Read the model definition and answer for the solid it produces. Units are mm, in the model's axes. Face numbers are marked on the shaded views. A direction names the side the tool comes from. Round coordinates to 2 decimals unless told otherwise and drop trailing zeros. Order: outer loops, then holes, each group sorted by start corner. A loop starts at its lowest first (then second) coordinate and runs counter-clockwise, first axis right, second up. Notation, with made-up numbers: (-15, 4) -> (3, 4) arc R12 ccw to (3, 8) -> close; hole circle Ø4 at (-38.75, 80). An arc over 180 degrees is marked (long way). One line per item, written item: value. Start each with the question number.
1. For the marked faces 1, 2 and 3, determine the directions among +Z, -Z, +X, -X, +Y, -Y from which every point of the face is accessible in a straight line to the end or side of a thin tool.
2. The mould has two halves that part along Y. Classify the marked faces 4, 5, 6 and 7: released by +Y, released by -Y, zero draft, split by the parting line, or undercut.
3. Section A-A (x = 14.5) is taken. Give the vertices of the cut face in (y, z), then the cut area to 3 significant figures.
4. Flat-ended cylindrical pins translate along their axes: pin 1 Ø1.2 at (y, z) = (0, 0) entering from -X; pin 2 Ø1 at (x, y) = (9.5, -2.5) entering from +Z; pin 3 Ø1.5 at (x, y) = (14, 3) entering from +Z. Find the tip coordinate at first contact, or state that the pin passes through.
5. Consider line 1 (Y direction, x = 9.5, z = 0.75); line 2 (Y direction, x = -6.15, z = 0) (3 decimals); line 3 (Y direction, x = 0, z = 0). Determine where each line is inside the solid, lowest interval first.
6. Section C-C (y = -6) is taken. Give the vertices of the cut face in (x, z), then the cut area to 3 significant figures.
7. Section D-D (z = -3.25) is taken. State how many separate pieces and enclosed holes the cut face has, then the cut area to 3 significant figures.
8. Section B-B (x = -3.75) is taken. Give the vertices of the cut face in (y, z) (3 decimals), then the cut area to 3 significant figures.
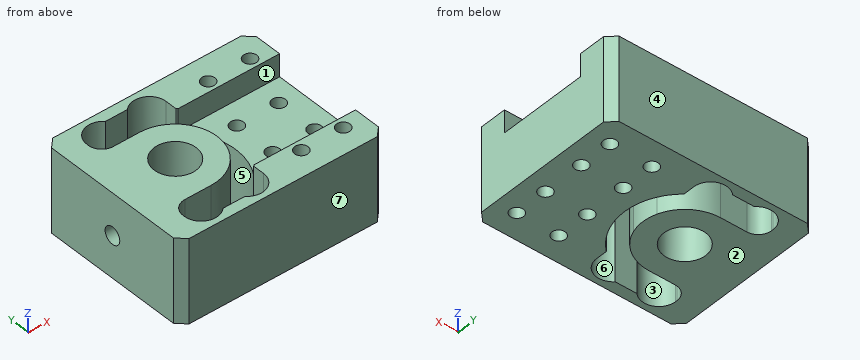
from build123d import *

# Parameters (mm, degrees)
SKETCH1_W                = 15
SKETCH1_H                = 19
BOSS_EXTRUDE1_DEPTH      = 5
BOSS_EXTRUDE1_DEPTH_BACK = 5
CUT_EXTRUDE1_START       = -6
SKETCH2_R                = 2
CUT_EXTRUDE1_DEPTH       = 16
SKETCH5_R                = 2
CUT_EXTRUDE4_DEPTH       = 17
CUT_EXTRUDE4_DEPTH_BACK  = 17
SKETCH6_R                = 2
CUT_EXTRUDE5_DEPTH       = 17
CUT_EXTRUDE5_DEPTH_BACK  = 17
SKETCH10_W               = 9.46
SKETCH10_H               = 13.6
CUT_EXTRUDE6_DEPTH       = 6
CUT_EXTRUDE6_DEPTH_BACK  = 6
BOSS_EXTRUDE2_START      = -5
SKETCH7_R                = 5
SKETCH7_R_2              = 2.5
BOSS_EXTRUDE2_DEPTH      = 10
BOSS_EXTRUDE3_DEPTH      = 5
FILLET1_R                = 1.6
SKETCH11_W               = 12.27
SKETCH11_H               = 19
BOSS_EXTRUDE4_DEPTH      = 10
CHAMFER1_SIZE            = 1
SKETCH16_W               = 5.80562201
SKETCH16_H               = 3.2
CUT_EXTRUDE8_DEPTH       = 11.5
CUT_EXTRUDE9_DEPTH       = 11.5
CUT_EXTRUDE10_DEPTH      = 2.7
TROU_TARAUD_M21_D        = 1.6
TROU_TARAUD_M2_51_D      = 2.05
TROU_TARAUD_M2_51_DEPTH  = 8.25
TROU_TARAUD_M2_51_TIP    = 0.615882135


with BuildPart() as part:
    # Sketch1 → Boss-Extrude1 (new body, two sides)
    with BuildSketch(Plane.XY) as boss_extrude1_sk:
        Rectangle(SKETCH1_W, SKETCH1_H)
    extrude(amount=BOSS_EXTRUDE1_DEPTH)
    extrude(boss_extrude1_sk.sketch, amount=-BOSS_EXTRUDE1_DEPTH_BACK)

    # Sketch2 → Cut-Extrude1 (cut)
    with BuildSketch(Plane.XY.offset(CUT_EXTRUDE1_START)):
        with Locations((-2.73, 6.8)):
            Circle(SKETCH2_R)
    cut_extrude1 = extrude(amount=CUT_EXTRUDE1_DEPTH, mode=Mode.SUBTRACT)

    # Mirror3: Cut-Extrude1 across plane
    add(cut_extrude1.mirror(Plane.ZX), mode=Mode.SUBTRACT)

    # Sketch5 → Cut-Extrude4 (cut, two sides)
    with BuildSketch(Plane.XY) as cut_extrude4_sk:
        with Locations((2.73, 6.8)):
            Circle(SKETCH5_R)
    extrude(amount=CUT_EXTRUDE4_DEPTH, mode=Mode.SUBTRACT)
    extrude(cut_extrude4_sk.sketch, amount=-CUT_EXTRUDE4_DEPTH_BACK, mode=Mode.SUBTRACT)

    # Sketch6 → Cut-Extrude5 (cut, two sides)
    with BuildSketch(Plane.XY) as cut_extrude5_sk:
        with Locations((2.73, -6.8)):
            Circle(SKETCH6_R)
    extrude(amount=CUT_EXTRUDE5_DEPTH, mode=Mode.SUBTRACT)
    extrude(cut_extrude5_sk.sketch, amount=-CUT_EXTRUDE5_DEPTH_BACK, mode=Mode.SUBTRACT)

    # Sketch10 → Cut-Extrude6 (cut, two sides)
    with BuildSketch(Plane.XY) as cut_extrude6_sk:
        Rectangle(SKETCH10_W, SKETCH10_H)
    extrude(amount=CUT_EXTRUDE6_DEPTH, mode=Mode.SUBTRACT)
    extrude(cut_extrude6_sk.sketch, amount=-CUT_EXTRUDE6_DEPTH_BACK, mode=Mode.SUBTRACT)



with BuildPart() as body_2:
    # Sketch7 → Boss-Extrude2 (new body)
    with BuildSketch(Plane.XY.offset(BOSS_EXTRUDE2_START)):
        Circle(SKETCH7_R)
        Circle(SKETCH7_R_2, mode=Mode.SUBTRACT)
    extrude(amount=BOSS_EXTRUDE2_DEPTH)


with BuildPart() as part_1:
    add(part.part)

    add(body_2.part)  # Boss-Extrude3 merges body 2
    # Sketch8 → Boss-Extrude3 (add, symmetric)
    with BuildSketch(Plane.XY):
        Polygon((0, 5), (-7.5, 5), (-7.5, 0), (-5, 0), align=None)
    boss_extrude3 = extrude(amount=BOSS_EXTRUDE3_DEPTH, both=True)

    # Mirror7: Boss-Extrude3 across plane
    add(boss_extrude3.mirror(Plane.ZX))

    # Fillet1
    fillet1_edges = [part_1.edges().sort_by_distance(p)[0] for p in [
        (-4.73, -5, 0),
        (-4.73, 5, 0),
    ]]
    fillet(fillet1_edges, radius=FILLET1_R)

    # Sketch11 → Boss-Extrude4 (add)
    with BuildSketch(Plane.XY.offset(5)):
        with Locations((10.865, 0)):
            Rectangle(SKETCH11_W, SKETCH11_H)
    extrude(amount=-BOSS_EXTRUDE4_DEPTH)

    # Chamfer1
    chamfer1_edges = [part_1.edges().sort_by_distance(p)[0] for p in [
        (17, 9.5, 0),
        (17, -9.5, 0),
        (-7.5, 9.5, 0),
        (-7.5, -9.5, 0),
    ]]
    chamfer(chamfer1_edges, length=CHAMFER1_SIZE)

    # Sketch16 → Cut-Extrude8 (cut)
    with BuildSketch(Plane.XY.offset(5)):
        with Locations((-0.227188995, 6.6)):
            Rectangle(SKETCH16_W, SKETCH16_H)
    cut_extrude8 = extrude(amount=-CUT_EXTRUDE8_DEPTH, mode=Mode.SUBTRACT)

    # Mirror8: Cut-Extrude8 across plane
    add(cut_extrude8.mirror(Plane.ZX), mode=Mode.SUBTRACT)

    # Sketch17 → Cut-Extrude9 (cut)
    with BuildSketch(Plane.XY.offset(5)):
        with BuildLine():
            ThreePointArc((2.678170763, -4.222250746), (5, 0), (2.678170763, 4.222250746))
            ThreePointArc((2.678170763, 4.222250746), (2.338473166, 5.740343478), (3.856565898, 6.080041075))
            ThreePointArc((3.856565898, 6.080041075), (7.2, 0), (3.856565898, -6.080041075))
            ThreePointArc((3.856565898, -6.080041075), (2.338473166, -5.740343478), (2.678170763, -4.222250746))
        make_face()
    extrude(amount=-CUT_EXTRUDE9_DEPTH, mode=Mode.SUBTRACT)

    # Sketch20 → Cut-Extrude10 (cut)
    with BuildSketch(Plane.XY.offset(5)):
        with BuildLine():
            Line((17, 5.3), (4.73, 5.3))
            ThreePointArc((4.73, 5.3), (7.103724375, 0), (4.73, -5.3))
            Line((4.73, -5.3), (17, -5.3))
            Line((17, -5.3), (17, 5.3))
        make_face()
    extrude(amount=-CUT_EXTRUDE10_DEPTH, mode=Mode.SUBTRACT)

    # Trou taraudé M21 (through all)
    with Locations(Plane.XY.offset(5)):
        with Locations((14.5, 2.5), (14.5, -2.5), (9.5, 2.5), (9.5, -2.5), (9.5, 6.5), (14.5, 6.5), (9.5, -6.5), (14.5, -6.5)):
            Hole(TROU_TARAUD_M21_D / 2)

    # Trou taraudé M2.51
    with Locations(Plane.ZY.offset(7.5)):
        with Locations((0, 0)):
            Hole(TROU_TARAUD_M2_51_D / 2, depth=TROU_TARAUD_M2_51_DEPTH)
            with Locations((0, 0, -(TROU_TARAUD_M2_51_DEPTH + TROU_TARAUD_M2_51_TIP / 2))):  # 118° drill point
                Cone(0, TROU_TARAUD_M2_51_D / 2, TROU_TARAUD_M2_51_TIP, mode=Mode.SUBTRACT)


solid = part_1.part
Answer:
1. face 1: +Z, +X
1. face 2: -Z, +X, -X, +Y, -Y
1. face 3: +Z, -Z
2. face 4: released by +Y
2. face 5: undercut
2. face 6: undercut
2. face 7: released by -Y
3. outline: (-9.5, -5) -> (-7.3, -5) -> (-7.3, 5) -> (-9.5, 5) -> close; (-5.7, -5) -> (-3.3, -5) -> (-3.3, 2.3) -> (-5.3, 2.3) -> (-5.3, 5) -> (-5.7, 5) -> close; (-1.7, -5) -> (1.7, -5) -> (1.7, 2.3) -> (-1.7, 2.3) -> close; (3.3, -5) -> (5.7, -5) -> (5.7, 5) -> (5.3, 5) -> (5.3, 2.3) -> (3.3, 2.3) -> close; (7.3, -5) -> (9.5, -5) -> (9.5, 5) -> (7.3, 5) -> close
3. area: 106 mm^2
4. pin 1: x = 2.43
4. pin 2: through
4. pin 3: z = 2.3
5. line 1: -9.5 to -7.3, -5.7 to -3.3, -1.7 to 1.7, 3.3 to 5.7, 7.3 to 9.5
5. line 2: -9.5 to -1.025, 1.025 to 9.5
5. line 3: -9.5 to -8.2, -5 to -2.5, 2.5 to 5, 8.2 to 9.5
6. outline: (-7.5, -5) -> (-4.61, -5) -> (-4.61, 5) -> (-7.5, 5) -> close; (4.73, -5) -> (8.88, -5) -> (8.88, 5) -> (4.73, 5) -> close; (10.12, -5) -> (13.88, -5) -> (13.88, 5) -> (10.12, 5) -> close; (15.12, -5) -> (17, -5) -> (17, 5) -> (15.12, 5) -> close
6. area: 127 mm^2
7. separate pieces: 1
7. enclosed holes: 10
7. area: 338 mm^2
8. outline: (-9.5, -5) -> (-8.52, -5) -> (-8.52, 5) -> (-9.5, 5) -> close; (-5.125, -5) -> (5.125, -5) -> (5.125, 5) -> (-5.125, 5) -> close; (8.52, -5) -> (9.5, -5) -> (9.5, 5) -> (8.52, 5) -> close; hole circle Ø2.05 at (0, 0)
8. area: 119 mm^2
